Read the model definition and answer for the solid it produces. Units are mm, in the model's axes. Face numbers are marked on the shaded views. Coordinates: 2 decimals unless noted, no trailing zeros. Write each loop counter-clockwise with the first axis right and the second up, starting at its lowest first coordinate (ties: lowest second). Pieces come first, ordered by that corner, then holes. Notation, with made-up numbers: (46, 11.25) - (97, 11.25) arc R19 cw to (97, 31.25) - close; hole circle Ø1 at (41, -25). An arc over 180 degrees is marked (long way). Use a Markdown table: item, result.
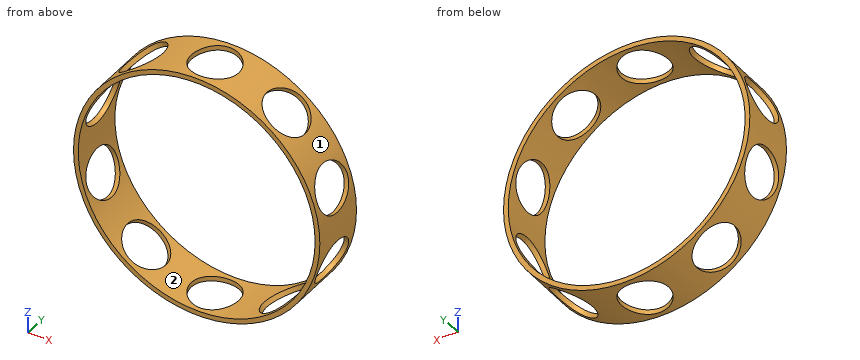
from build123d import *

# Parameters (mm, degrees)
SKETCH1_R           = 13
SKETCH1_R_2         = 12.5
BOSS_EXTRUDE2_DEPTH = 6
SKETCH5_R           = 2.5
CUT_EXTRUDE1_DEPTH  = 14
CIRPATTERN1_COUNT   = 5


with BuildPart() as part:
    # Sketch1 → Boss-Extrude2 (new body)
    with BuildSketch(Plane(origin=(0, 0, 0), x_dir=(1, 0, 0), z_dir=(0, 1, 0))):
        Circle(SKETCH1_R)
        Circle(SKETCH1_R_2, mode=Mode.SUBTRACT)
    extrude(amount=BOSS_EXTRUDE2_DEPTH)

    # Sketch5 → Cut-Extrude1 (cut, symmetric)
    with BuildSketch(Plane.XY):
        with Locations((0, 3)):
            Circle(SKETCH5_R)
    cut_extrude1 = extrude(amount=CUT_EXTRUDE1_DEPTH, both=True, mode=Mode.SUBTRACT)

    # CirPattern1: Cut-Extrude1 ×5 about axis
    cirpattern1_axis = Axis((0, 6, 0), (0, -1, 0))
    for i in range(1, CIRPATTERN1_COUNT):
        add(cut_extrude1.rotate(cirpattern1_axis, i * 360 / CIRPATTERN1_COUNT), mode=Mode.SUBTRACT)


solid = part.part
(1) A cutting plane is placed at A-A, the plane z = 0. Write down the section's boundary in (x, y), and give its area (3 significant figures).
Report:
| item | result |
|---|---|
| outline | (-13, 0) - (-12.5, 0) - (-12.5, 6) - (-13, 6) - close; (12.5, 0) - (13, 0) - (13, 6) - (12.5, 6) - close |
| area | 6.00 mm² |
(2) A cutting plane is placed at B-B, the plane x = 0. Write down the section's boundary in (y, z), and give its area (4 significant figures).
Report:
| item | result |
|---|---|
| outline | (0, -13) - (0.5, -13) - (0.5, -12.5) - (0, -12.5) - close; (0, 12.5) - (0.5, 12.5) - (0.5, 13) - (0, 13) - close; (5.5, -13) - (6, -13) - (6, -12.5) - (5.5, -12.5) - close; (5.5, 12.5) - (6, 12.5) - (6, 13) - (5.5, 13) - close |
| area | 1.000 mm² |
(3) The mould has two halves that part along Z. Classify the marked faces 1 and 2: pulls with the +Z half, pulls with the -Z half, needs draft (parallel to the pull), parting line crosses it, or undercut.
Report:
| item | result |
|---|---|
| face 1 | parting line crosses it |
| face 2 | undercut |
(4) Each of these flat-tipped pins is pushed along its axis until it touches: P1, Ø1.5, axis at y = 4.5, z = -5.5, coming from the -X side; P2, Ø3, axis at x = 8.5, y = 1.5, coming from the +Z side (3 decimals); P3, Ø1.5, axis at x = 3, y = 3.5, coming from the -Z side; P4, Ø3, axis at x = 0, y = 3, coming from the -Z side. Where does it stop, or does it pass through?
Report:
| item | result |
|---|---|
| P1 | stops at x = -11.93 |
| P2 | stops at z = 10.715 |
| P3 | stops at z = -12.79 |
| P4 | passes through |
(5) Straight lines are drawn through the part: L1, parallel to Y at x = 0, z = 12.8; L2, parallel to X at y = 3, z = 0; L3, parallel to X at y = 0.5, z = 5. For each, find the intervals that lie inside material, in ascending order.
Report:
| item | result |
|---|---|
| L1 | y = 0 to 0.5, 5.5 to 6 |
| L2 | x = -13 to -12.5, 12.5 to 13 |
| L3 | x = -12 to -11.46, 11.46 to 12 |
(6) A cutting plane is placed at C-C, the plane y = 4. Count the separate pieces of the cut face and the enclosed holes in it, and give its area (3 significant figures).
Report:
| item | result |
|---|---|
| separate pieces | 10 |
| enclosed holes | 0 |
| area | 17.0 mm² |
